```python
from build123d import *

# Parameters (mm, degrees)
SKETCH_1_R          = 15
SKETCH_1_R_2        = 1.5
EXTRUDE_1_DEPTH     = 3
SKETCH_2_R          = 5.035
SKETCH_2_R_2        = 0.8
EXTRUDE_2_DEPTH     = 4.4
SKETCH_4_R          = 5.535
EXTRUDE_3_DEPTH     = 0.2
CHAMFER_1_SIZE      = 0.5
CHAMFER_3_SIZE      = 0.5
CHAMFER_4_SIZE      = 1.6
CUT_EXTRUDE_START   = -10
SKETCH_5_R          = 0.8
CUT_EXTRUDE_1_DEPTH = 10


with BuildPart() as part:
    # 草图1 → 凸台-拉伸1 (new body)
    with BuildSketch(Plane(origin=(0, 0, 0), x_dir=(1, 0, 0), z_dir=(0, 1, 0))):
        with Locations(Location((0, 0, 0), (0, 0, 270))):
            Circle(SKETCH_1_R)
        with Locations(Location((0, 10, 0), (0, 0, 270))):
            Circle(SKETCH_1_R_2, mode=Mode.SUBTRACT)
        with Locations(Location((10, 0, 0), (0, 0, 270))):
            Circle(SKETCH_1_R_2, mode=Mode.SUBTRACT)
        with Locations(Location((0, -10, 0), (0, 0, 270))):
            Circle(SKETCH_1_R_2, mode=Mode.SUBTRACT)
        with Locations(Location((-10, 0, 0), (0, 0, 270))):
            Circle(SKETCH_1_R_2, mode=Mode.SUBTRACT)
    extrude(amount=EXTRUDE_1_DEPTH)

    # 草图2 → 凸台-拉伸2 (add)
    with BuildSketch(Plane(origin=(0, 3, 0), x_dir=(1, 0, 0), z_dir=(0, 1, 0))):
        with Locations(Location((0, 0, 0), (0, 0, 270))):
            Circle(SKETCH_2_R)
        with Locations(Location((2, 0, 0), (0, 0, 270))):
            Circle(SKETCH_2_R_2, mode=Mode.SUBTRACT)
        with Locations(Location((-2, 0, 0), (0, 0, 90))):
            Circle(SKETCH_2_R_2, mode=Mode.SUBTRACT)
    extrude(amount=EXTRUDE_2_DEPTH)

    # 草图4 → 凸台-拉伸3 (add)
    with BuildSketch(Plane(origin=(0, 3, 0), x_dir=(1, 0, 0), z_dir=(0, 1, 0))):
        with Locations(Location((0, 0, 0), (0, 0, 270))):
            Circle(SKETCH_4_R)
    extrude(amount=EXTRUDE_3_DEPTH)

    # 倒角1
    chamfer_1_edges = [part.edges().sort_by_distance(p)[0] for p in [
        (0, 7.4, -5.035),
    ]]
    chamfer(chamfer_1_edges, length=CHAMFER_1_SIZE)

    # 倒角3
    chamfer_3_edges = [part.edges().sort_by_distance(p)[0] for p in [
        (0, 0, -15),
        (0, 3, -15),
    ]]
    chamfer(chamfer_3_edges, length=CHAMFER_3_SIZE)

    # 倒角4
    chamfer_4_edges = [part.edges().sort_by_distance(p)[0] for p in [
        (0, 3, 8.5),
        (-10, 3, -1.5),
        (0, 3, -11.5),
        (10, 3, -1.5),
    ]]
    chamfer(chamfer_4_edges, length=CHAMFER_4_SIZE)

    # 草图5 → 切除-拉伸1 (cut)
    with BuildSketch(Plane(origin=(0, 7.4, 0), x_dir=(1, 0, 0), z_dir=(0, 1, 0)).offset(CUT_EXTRUDE_START)):
        with Locations(Location((2, 0, 0), (0, 0, 270))):
            Circle(SKETCH_5_R)
        with Locations(Location((-2, 0, 0), (0, 0, 90))):
            Circle(SKETCH_5_R)
    extrude(amount=CUT_EXTRUDE_1_DEPTH, mode=Mode.SUBTRACT)


solid = part.part
```
Build history of the part. All positions in model axes, mm. Coordinates: 2 decimals unless noted, no trailing zeros. Order: outer loops, then holes, each group sorted by start corner. A loop starts at its lowest first (then second) coordinate and runs counter-clockwise, first axis right, second up.
Item 1: Saw through at D-D on y = 4.5. List the corners of the cut face in (x, z) (3 decimals), then the cut area to 3 significant figures.
Filled in:
outline: circle Ø10.07 at (0, 0); hole circle Ø1.6 at (-2, 0); hole circle Ø1.6 at (2, 0)
area: 75.6 mm2
Item 2: Drop flat-ended pins along their axis: pin 1 Ø4 at (x, z) = (-10, 0) entering from +Y; pin 2 Ø8 at (x, z) = (5.5, 10) entering from +Y; pin 3 Ø2.5 at (x, z) = (10, 0) entering from +Y; pin 4 Ø4 at (x, z) = (-3.5, 6) entering from +Y. Give the stop position or say it passes through.
Filled in:
pin 1: stops at y = 1.9
pin 2: stops at y = 3
pin 3: passes through
pin 4: stops at y = 6.99
Item 3: Drill centre lines: L1, parallel to X at y = 5.5, z = 0 (3 decimals); L2, parallel to X at y = 0.8, z = 0; L3, parallel to X at y = 1.75, z = 0.5. Where is each one in solid material? Low to high.
Filled in:
L1: x = -5.035 to -2.8, -1.2 to 1.2, 2.8 to 5.035
L2: x = -15 to -11.5, -8.5 to -2.8, -1.2 to 1.2, 2.8 to 8.5, 11.5 to 15
L3: x = -14.99 to -11.78, -8.22 to -2.62, -1.38 to 1.38, 2.62 to 8.22, 11.78 to 14.99
Item 4: Saw through at A-A on x = 0. State how many separate pieces and enclosed holes the cut face has, then the cut area to 3 significant figures.
Filled in:
separate pieces: 3
enclosed holes: 0
area: 111 mm2
Item 5: Saw through at B-B on y = 2. List the corners of the cut face in (x, z).
Filled in:
outline: circle Ø30 at (0, 0); hole circle Ø4.2 at (-10, 0); hole circle Ø1.6 at (-2, 0); hole circle Ø4.2 at (0, -10); hole circle Ø4.2 at (0, 10); hole circle Ø1.6 at (2, 0); hole circle Ø4.2 at (10, 0)
Item 6: Mould opens along X. For faces 1 (the cylindrical face through (1.512, 5.024, 4.802)), 2 (the cylindrical face through (8.536, 0.69, -0.325)), 3 (the flat face through (0, 3, 6)) say: released by +X, released by -X, zero draft, split by the parting line, or undercut.
Filled in:
face 1: split by the parting line
face 2: undercut
face 3: zero draft
